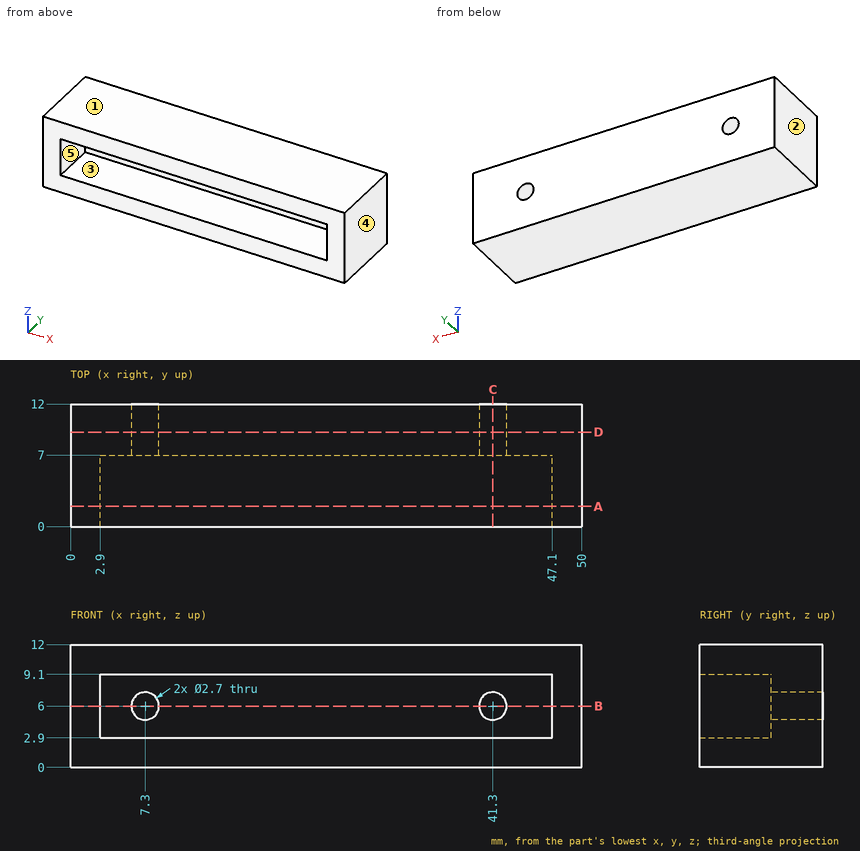
Answer from the drawing. Dimensions are ordinates in mm from the lowest x, y and z of the part. A direction names the side the tool comes from. Give positions to 0.01 mm unless a question says otherwise; leave off trailing zeros. Write each loop counter-clockwise with the first axis right and the second up, starting at its lowest first coordinate (ties: lowest second). Pieces come first, ordered by that corner, then holes. Notation, with made-up numbers: (36, 21.5) - (54, 21.5) arc R22 ccw to (54, 46.5) - close; hole circle Ø4 at (53, -26). An arc over 180 degrees is marked (long way). Answer in a Markdown table with one row per item. Add a question column.
Item 1: Section B-B, the plane z = 6 is taken. Write down the section's boundary in (x, y), and give its area (3 significant figures).
Item 2: A tool of negligible diameter and unlimited length cuts with its end or side. For the marked faces 4 and 5, from which of +Z, -Z, +X, -X, +Y, -Y can it reach the whole face along a straight path? Write none if from no direction.
Item 3: Section A-A, the plane y = 2 is taken. Write down the section's boundary in (x, z), and give its area (3 significant figures).
Item 4: Section C-C, the plane x = 41.3 is taken. Write down the section's boundary in (y, z).
Item 5: Determine the mould class of the marked faces 1, 2 and 3 for opening direction Z: pulls with the +Z half, pulls with the -Z half, needs draft (parallel to the pull), parting line crosses it, or undercut.
Item 6: Flat-ended cylindrical pins translate along their axes: P1, Ø1, axis at x = 27, y = 9, coming from the -Z side; P2, Ø5, axis at x = 35, z = 6, coming from the -Y side. Find the tip coordinate at first contact, or state that the pin passes through.
Item 7: Section D-D, the plane y = 9.25 is taken. Write down the section's boundary in (x, z), and give its area (3 significant figures).
Item 8: Find the intervals of material crossed by L1, parallel to Z at x = 42, y = 5.75; L2, parallel to X at y = 10, z = 7; L3, parallel to Z at x = 41.3, y = 9.15, in increasing order.
Recorded:
| question | item | result |
|---|---|---|
| 1 | outline | (0, 0) - (2.9, 0) - (2.9, 7) - (5.95, 7) - (5.95, 12) - (0, 12) - close; (8.65, 7) - (39.95, 7) - (39.95, 12) - (8.65, 12) - close; (42.65, 7) - (47.1, 7) - (47.1, 0) - (50, 0) - (50, 12) - (42.65, 12) - close |
| 1 | area | 264 mm2 |
| 2 | face 4 | +Z, -Z, +X, +Y, -Y |
| 2 | face 5 | -Y |
| 3 | outline | (0, 0) - (50, 0) - (50, 12) - (0, 12) - close; hole (2.9, 2.9) - (47.1, 2.9) - (47.1, 9.1) - (2.9, 9.1) - close |
| 3 | area | 326 mm2 |
| 4 | outline | (0, 0) - (12, 0) - (12, 4.65) - (7, 4.65) - (7, 2.9) - (0, 2.9) - close; (0, 9.1) - (7, 9.1) - (7, 7.35) - (12, 7.35) - (12, 12) - (0, 12) - close |
| 5 | face 1 | pulls with the +Z half |
| 5 | face 2 | needs draft |
| 5 | face 3 | undercut |
| 6 | P1 | stops at z = 0 |
| 6 | P2 | stops at y = 7 |
| 7 | outline | (0, 0) - (50, 0) - (50, 12) - (0, 12) - close; hole circle Ø2.7 at (7.3, 6); hole circle Ø2.7 at (41.3, 6) |
| 7 | area | 589 mm2 |
| 8 | L1 | z = 0 to 2.9, 9.1 to 12 |
| 8 | L2 | x = 0 to 6.39, 8.21 to 40.39, 42.21 to 50 |
| 8 | L3 | z = 0 to 4.65, 7.35 to 12 |
